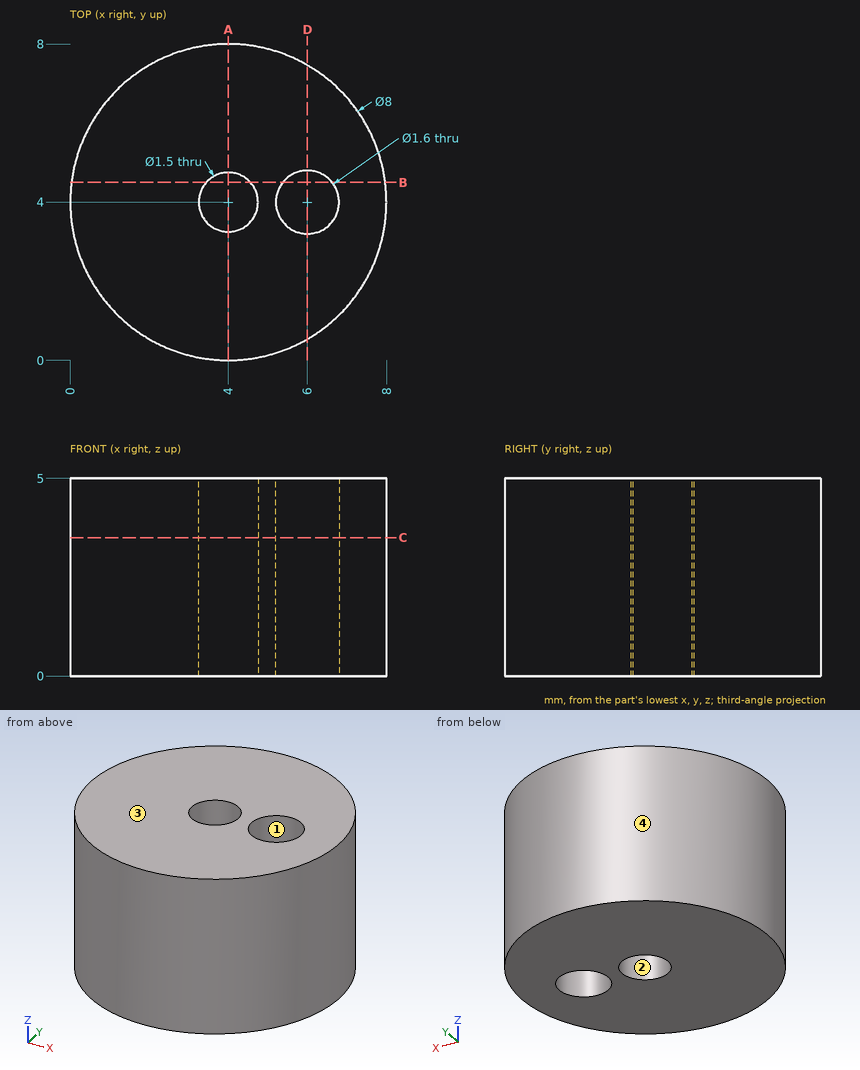
Geometry check sheet. Reference: drawing and pictorial views, mm from the part's lowest x, y, z. Round coordinates to 2 decimals unless told otherwise and drop trailing zeros. Loops run counter-clockwise (first coordinate to the right, second up) from the corner with the lowest first, then second, coordinate; pieces in that order, holes last. Notation, with made-up numbers: (57.5, -32.75) -> (63.5, -32.75) arc R17 cw to (63.5, 0.25) -> close; hole circle Ø8 at (3.5, -21). An arc over 180 degrees is marked (long way). Answer as a JSON object with one key per item and string values. Group by question number.
Item 1: Depth check by flat-ended pin: pin 1 Ø1.2 at (x, y) = (4, 4) entering from +Z; pin 2 Ø1.5 at (x, z) = (2, 2.5) entering from -Y; pin 3 Ø3 at (x, z) = (6.5, 3) entering from -Y. Enter the tip coordinate at first touch or a pass-through.
Item 2: Release check for a two-part mould opening along X. For the marked faces 1, 2, 3 and 4 record: pulls with the +X half, pulls with the -X half, needs draft (parallel to the pull), parting line crosses it, or undercut.
Item 3: Thickness scan on line 1 along Y through (x, z) = (4, 1.9); line 2 along Y through (x, z) = (4.5, 3.05); line 3 along X through (y, z) = (7.5, 2.75). Record the ranges inside material, lowest first.
Item 4: Cross-section at D-D, the plane x = 6. Record the cut outline in (y, z).
Item 5: Cross-section at C-C, the plane z = 3.5. Record the cut outline in (x, y).
Item 6: Cross-section at A-A, the plane x = 4. Record the cut outline in (y, z).
Item 7: Cross-section at B-B, the plane y = 4.5. Record the cut outline in (x, z), plus the area to 3 significant figures.
Determined:
{
 "1": {"pin 1": "passes through", "pin 2": "stops at y = 0.2", "pin 3": "stops at y = 0.13"},
 "2": {"face 1": "undercut", "face 2": "undercut", "face 3": "needs draft", "face 4": "parting line crosses it"},
 "3": {"line 1": "y = 0 to 3.25, 4.75 to 8", "line 2": "y = 0.03 to 3.44, 4.56 to 7.97", "line 3": "x = 2.06 to 5.94"},
 "4": {"outline": "(0.54, 0) -> (3.2, 0) -> (3.2, 5) -> (0.54, 5) -> close; (4.8, 0) -> (7.46, 0) -> (7.46, 5) -> (4.8, 5) -> close"},
 "5": {"outline": "circle Ø8 at (4, 4); hole circle Ø1.5 at (4, 4); hole circle Ø1.6 at (6, 4)"},
 "6": {"outline": "(0, 0) -> (3.25, 0) -> (3.25, 5) -> (0, 5) -> close; (4.75, 0) -> (8, 0) -> (8, 5) -> (4.75, 5) -> close"},
 "7": {"outline": "(0.03, 0) -> (3.44, 0) -> (3.44, 5) -> (0.03, 5) -> close; (4.56, 0) -> (5.38, 0) -> (5.38, 5) -> (4.56, 5) -> close; (6.62, 0) -> (7.97, 0) -> (7.97, 5) -> (6.62, 5) -> close", "area": "27.9 mm²"}
}
